```python
from build123d import *

# Parameters (mm, degrees)
SKETCH1_R           = 2.55
BOSS_EXTRUDE1_DEPTH = 15
BOSS_EXTRUDE2_DEPTH = 100
CUT_EXTRUDE1_REACH  = 188.053
SKETCH3_R           = 7.5
SKETCH3_R_2         = 3.5


with BuildPart() as part:
    # Sketch1 → Boss-Extrude1 (new body)
    with BuildSketch(Plane(origin=(0, 0, 0), x_dir=(1, 0, 0), z_dir=(0, 1, 0))):
        Polygon((-65.40737726, 35.40737726), (-65.40737726, 65.40737726), (-35.40737726, 65.40737726), (35.40737726, 65.40737726), (65.40737726, 65.40737726), (65.40737726, 35.40737726), (65.40737726, -35.40737726), (65.40737726, -65.40737726), (35.40737726, -65.40737726), (-35.40737726, -65.40737726), (-65.40737726, -65.40737726), (-65.40737726, -35.40737726), align=None)
        with Locations(Location((37.759502115, 37.759502115, 0), (0, 0, 270))):
            Circle(SKETCH1_R, mode=Mode.SUBTRACT)
        with Locations(Location((37.759502115, -37.759502115, 0), (0, 0, 270))):
            Circle(SKETCH1_R, mode=Mode.SUBTRACT)
        with Locations(Location((-37.759502115, -37.759502115, 0), (0, 0, 270))):
            Circle(SKETCH1_R, mode=Mode.SUBTRACT)
        with Locations(Location((-37.759502115, 37.759502115, 0), (0, 0, 270))):
            Circle(SKETCH1_R, mode=Mode.SUBTRACT)
    extrude(amount=BOSS_EXTRUDE1_DEPTH)

    # Sketch2 → Boss-Extrude2 (add)
    with BuildSketch(Plane(origin=(0, 15, 0), x_dir=(1, 0, 0), z_dir=(0, 1, 0))):
        Polygon((50.40737726, -50.40737726), (50.40737726, -65.40737726), (65.40737726, -65.40737726), (65.40737726, 65.40737726), (50.40737726, 65.40737726), (50.40737726, 50.40737726), align=None)
        Polygon((-65.40737726, 65.40737726), (-65.40737726, -65.40737726), (-50.40737726, -65.40737726), (-50.40737726, -50.40737726), (-50.40737726, 50.40737726), (-50.40737726, 65.40737726), align=None)
    extrude(amount=BOSS_EXTRUDE2_DEPTH)

    # Cut-Extrude1: up to this face of the body (flat: up to its plane)
    cut_extrude1_end = Plane(part.part.faces().sort_by_distance((65.40737726, 57.5, 0))[0])
    # Sketch3 → Cut-Extrude1 (cut, up to the picked face)
    with BuildSketch(Plane.ZY.offset(65.40737726), mode=Mode.PRIVATE) as cut_extrude1_sk1:
        with Locations((32.70368863, 86.25)):
            Circle(SKETCH3_R)
    cut_extrude1_tool1 = split(extrude(cut_extrude1_sk1.sketch, amount=-CUT_EXTRUDE1_REACH, mode=Mode.PRIVATE), bisect_by=cut_extrude1_end, keep=Keep.BOTH, mode=Mode.PRIVATE)
    # Sketch3 → Cut-Extrude1 (cut, up to the picked face)
    with BuildSketch(Plane.ZY.offset(65.40737726), mode=Mode.PRIVATE) as cut_extrude1_sk2:
        with Locations((14.678572243, 70.404016937)):
            Circle(SKETCH3_R_2)
    cut_extrude1_tool2 = split(extrude(cut_extrude1_sk2.sketch, amount=-CUT_EXTRUDE1_REACH, mode=Mode.PRIVATE), bisect_by=cut_extrude1_end, keep=Keep.BOTH, mode=Mode.PRIVATE)
    # Sketch3 → Cut-Extrude1 (cut, up to the picked face)
    with BuildSketch(Plane.ZY.offset(65.40737726), mode=Mode.PRIVATE) as cut_extrude1_sk3:
        with Locations((50.728805017, 102.095983063)):
            Circle(SKETCH3_R_2)
    cut_extrude1_tool3 = split(extrude(cut_extrude1_sk3.sketch, amount=-CUT_EXTRUDE1_REACH, mode=Mode.PRIVATE), bisect_by=cut_extrude1_end, keep=Keep.BOTH, mode=Mode.PRIVATE)
    add(cut_extrude1_tool1.solids().sort_by(Axis((-65.407377, 86.25, 32.703689), (1, 0, 0)))[0], mode=Mode.SUBTRACT)
    add(cut_extrude1_tool2.solids().sort_by(Axis((-65.407377, 70.404017, 14.678572), (1, 0, 0)))[0], mode=Mode.SUBTRACT)
    add(cut_extrude1_tool3.solids().sort_by(Axis((-65.407377, 102.095983, 50.728805), (1, 0, 0)))[0], mode=Mode.SUBTRACT)


solid = part.part
```
Design review of the part built by this model. Coordinates are the model's own, in mm. A direction names the side the tool comes from. Coordinates: 2 decimals unless noted, no trailing zeros. Order: outer loops, then holes, each group sorted by start corner. A loop starts at its lowest first (then second) coordinate and runs counter-clockwise, first axis right, second up. Notation, with made-up numbers: (5, 77) -> (46, 77) arc R6 ccw to (46, 84) -> close; hole circle Ø2 at (-20, 77.5). An arc over 180 degrees is marked (long way). One line per item, written item: value. Start each with the question number.
Q1. Insertion check: pin 1 Ø8 at (y, z) = (102.1, 50.73) entering from -X; pin 2 Ø6.5 at (x, z) = (-37.76, 37.76) entering from +Y. Each pin has a flat end and moves straight along its axis. Give the tip position at first contact, or say it passes through.
Q2. Take a section at C-C, the plane y = 52.5. State the section outline as (x, z) points.
Q3. Take a section at B-B, the plane z = -12. State the section outline as (x, y) points.
Q4. For probe 1 along X at (y, z) = (96, 36); probe 2 along Y at (x, z) = (42, -50.5); probe 3 along Y at (x, z) = (-57, 35.5), list the stretches that pass through material, from the lowest coordinate up.
Q5. Take a section at A-A, the plane y = 86.25. State the section outline as (x, z) points.
Q6. Tool access review of faces 1 (the cylindrical face through (39.48, 7.4, 35.88)), 2 (the flat face through (50.407, 64, -1)): name each direction out of +Z, -Z, +X, -X, +Y, -Y from which nothing blocks a thin tool from reaching the whole face with its end or side.
Q7. Mouldability with a two-part tool opening along Z and no side actions: class faces 3 (the flat face through (65.407, 57, 1)), 4 (the flat face through (-0.3, 14.6, 65.407)), 5 (the cylindrical face through (57.802, 79.596, 36.164)) as pulls with the +Z half, pulls with the -Z half, needs draft (parallel to the pull), parting line crosses it, or undercut.
Q8. Take a section at D-D, the plane x = 57.5. State the section outline as (y, z) points, then the cut area to 3 significant figures.
Values follow:
1. pin 1: stops at x = -65.41
1. pin 2: stops at y = 15
2. outline: (-65.41, -65.41) -> (-50.41, -65.41) -> (-50.41, 65.41) -> (-65.41, 65.41) -> close; (50.41, -65.41) -> (65.41, -65.41) -> (65.41, 65.41) -> (50.41, 65.41) -> close
3. outline: (-65.41, 0) -> (65.41, 0) -> (65.41, 115) -> (50.41, 115) -> (50.41, 15) -> (-50.41, 15) -> (-50.41, 115) -> (-65.41, 115) -> close
4. probe 1: x = -65.41 to -50.41, 50.41 to 65.41
4. probe 2: y = 0 to 15
4. probe 3: y = 0 to 79.29, 93.21 to 115
5. outline: (-65.41, -65.41) -> (-50.41, -65.41) -> (-50.41, 25.2) -> (-65.41, 25.2) -> close; (-65.41, 40.2) -> (-50.41, 40.2) -> (-50.41, 65.41) -> (-65.41, 65.41) -> close; (50.41, -65.41) -> (65.41, -65.41) -> (65.41, 25.2) -> (50.41, 25.2) -> close; (50.41, 40.2) -> (65.41, 40.2) -> (65.41, 65.41) -> (50.41, 65.41) -> close
6. face 1: +Y, -Y
6. face 2: +Z, -Z, +Y
7. face 3: needs draft
7. face 4: pulls with the +Z half
7. face 5: undercut
8. outline: (0, -65.41) -> (115, -65.41) -> (115, 65.41) -> (0, 65.41) -> close; hole circle Ø7 at (70.4, 14.68); hole circle Ø15 at (86.25, 32.7); hole circle Ø7 at (102.1, 50.73)
8. area: 14,800 mm2
